```python
from build123d import *

# Parameters (mm, degrees)
SKETCH_2_W                     = 4.9
SKETCH_2_H                     = 7
EXTRUDE_1_DEPTH                = 2.7
EXTRUDE_2_DEPTH                = 0.25
FILLET_1_R                     = 0.05
CHAMFER_1_SIZE                 = 0.4
PATTERN_LINEAR_2_COUNT         = 2
PATTERN_LINEAR_2_PITCH         = 2.5
FILLET_1_OF_PATTERN_LINEAR_2_R = 0.05
MIRROR_START                   = -1.5
MIRROR_1_DEPTH                 = 0.5
MIRROR_START_2                 = 1
MIRROR_1_2_DEPTH               = 0.5
CHAMFER_2_SIZE                 = 0.4
CHAMFER_3_SIZE                 = 0.15
CHAMFER_3_SIZE2                = 0.649721381
CHAMFER_4_SIZE                 = 0.15
CHAMFER_4_SIZE2                = 0.649721381
SKETCH_7_R                     = 0.15
CUT_EXTRUDE_2_DEPTH            = 0.02
MOVE_BODY_2_ANGLE              = 120


with BuildPart() as part:
    # Эскиз2 → Бобышка-Вытянуть1 (new body)
    with BuildSketch(Plane(origin=(0, 0.15, 0), x_dir=(-1, 0, 0), z_dir=(0, 1, 0))):
        Rectangle(SKETCH_2_W, SKETCH_2_H)
    extrude(amount=EXTRUDE_1_DEPTH)

    # Эскиз4 → Вытянуть-Тонкостенный2 (add, symmetric)
    with BuildSketch(Plane(origin=(1.25, 0, 0), x_dir=(0, 0, -1), z_dir=(1, 0, 0))):
        with BuildLine():
            Line((-3.5, 1.3), (-3.905923723, 1.3))
            ThreePointArc((-3.905923723, 1.3), (-4.063504056, 1.223160215), (-4.1, 1.051684386))
            Line((-4.1, 1.051684386), (-3.9, 0.248315614))
            ThreePointArc((-3.9, 0.248315614), (-3.936495944, 0.076839785), (-4.094076277, 0))
            Line((-4.094076277, 0), (-4.6, 0))
            Line((-4.6, 0), (-4.6, 0.35))
            Line((-4.6, 0.35), (-4.285997426, 0.35))
            Line((-4.285997426, 0.35), (-4.439633485, 0.967132062))
            ThreePointArc((-4.439633485, 0.967132062), (-4.339269639, 1.438690592), (-3.905923723, 1.65))
            Line((-3.905923723, 1.65), (-3.5, 1.65))
            Line((-3.5, 1.65), (-3.5, 1.3))
        make_face()
    extrude_2 = extrude(amount=EXTRUDE_2_DEPTH, both=True)

    # Скругление1
    fillet_1_edges = [part.edges().sort_by_distance(p)[0] for p in [
        (1.25, 0.35, 4.285997426),
    ]]
    fillet(fillet_1_edges, radius=FILLET_1_R)

    # Фаска1
    chamfer_1_edges = [part.edges().sort_by_distance(p)[0] for p in [
        (0, 2.85, 3.5),
    ]]
    chamfer(chamfer_1_edges, length=CHAMFER_1_SIZE)

    # Линейный массив2: Вытянуть-Тонкостенный2 ×2
    with Locations(*[(-i * PATTERN_LINEAR_2_PITCH, 0, 0) for i in range(1, PATTERN_LINEAR_2_COUNT)]):
        add(extrude_2)

    # Скругление1 of Линейный массив2
    fillet_1_of_pattern_linear_2_edges = [part.edges().sort_by_distance(p)[0] for p in [
        (-1.25, 0.35, 4.285997426),
    ]]
    fillet(fillet_1_of_pattern_linear_2_edges, radius=FILLET_1_OF_PATTERN_LINEAR_2_R)

    # Зеркальное отражение1: read off the stored shape, not the designer's step
    # Зеркальное отражение1 outline → Зеркальное отражение1 (add)
    with BuildSketch(Plane.YZ.offset(MIRROR_START)):
        with BuildLine():
            Line((0, -4.6), (0.35, -4.6))
            Line((0.35, -4.6), (0.35, -4.349971142))
            ThreePointArc((0.35, -4.349971142), (0.369209946, -4.310576059), (0.412078903, -4.301452073))
            Line((0.412078903, -4.301452073), (0.967132062, -4.439633485))
            ThreePointArc((0.967132062, -4.439633485), (1.438690592, -4.339269639), (1.65, -3.905923723))
            Line((1.65, -3.905923723), (1.65, -3.5))
            Line((1.65, -3.5), (1.3, -3.5))
            Line((1.3, -3.5), (1.3, -3.905923723))
            ThreePointArc((1.3, -3.905923723), (1.223160215, -4.063504056), (1.051684386, -4.1))
            Line((1.051684386, -4.1), (0.248315614, -3.9))
            ThreePointArc((0.248315614, -3.9), (0.076839785, -3.936495944), (0, -4.094076277))
            Line((0, -4.094076277), (0, -4.6))
        make_face()
    extrude(amount=MIRROR_1_DEPTH)

    # Mirror 1 2 outline → Mirror 1 2 (add)
    with BuildSketch(Plane.YZ.offset(MIRROR_START_2)):
        with BuildLine():
            Line((0, -4.6), (0.35, -4.6))
            Line((0.35, -4.6), (0.35, -4.349971142))
            ThreePointArc((0.35, -4.349971142), (0.369209946, -4.310576059), (0.412078903, -4.301452073))
            Line((0.412078903, -4.301452073), (0.967132062, -4.439633485))
            ThreePointArc((0.967132062, -4.439633485), (1.438690592, -4.339269639), (1.65, -3.905923723))
            Line((1.65, -3.905923723), (1.65, -3.5))
            Line((1.65, -3.5), (1.3, -3.5))
            Line((1.3, -3.5), (1.3, -3.905923723))
            ThreePointArc((1.3, -3.905923723), (1.223160215, -4.063504056), (1.051684386, -4.1))
            Line((1.051684386, -4.1), (0.248315614, -3.9))
            ThreePointArc((0.248315614, -3.9), (0.076839785, -3.936495944), (0, -4.094076277))
            Line((0, -4.094076277), (0, -4.6))
        make_face()
    extrude(amount=MIRROR_1_2_DEPTH)

    # Фаска2
    chamfer_2_edges = [part.edges().sort_by_distance(p)[0] for p in [
        (0, 2.85, -3.5),
    ]]
    chamfer(chamfer_2_edges, length=CHAMFER_2_SIZE)

    # Фаска3
    chamfer_3_edges = [part.edges().sort_by_distance(p)[0] for p in [
        (0, 0.15, -3.5),
    ]]
    chamfer_3_side = [part.faces().sort_by_distance(p)[0] for p in [
        (0, 0.15, 0),
    ]]
    chamfer(chamfer_3_edges, length=CHAMFER_3_SIZE, length2=CHAMFER_3_SIZE2, reference=chamfer_3_side[0])

    # Фаска4
    chamfer_4_edges = [part.edges().sort_by_distance(p)[0] for p in [
        (0, 0.15, 3.5),
    ]]
    chamfer_4_side = [part.faces().sort_by_distance(p)[0] for p in [
        (0, 0.15, 0.075),
    ]]
    chamfer(chamfer_4_edges, length=CHAMFER_4_SIZE, length2=CHAMFER_4_SIZE2, reference=chamfer_4_side[0])

    # Эскиз7 → Вырез-Вытянуть2 (cut)
    with BuildSketch(Plane(origin=(0, 2.85, 0), x_dir=(1, 0, 0), z_dir=(0, 1, 0))):
        with Locations(Location((-1.95, -2.8, 0), (0, 0, 270))):
            Circle(SKETCH_7_R)
    extrude(amount=-CUT_EXTRUDE_2_DEPTH, mode=Mode.SUBTRACT)


with BuildPart() as part_1:
    # Move Body 2: read off the stored shape, not the designer's step
    # Move Body 2: moved
    add(part.part.moved(Location((1.25, 0, -4.425))).rotate(Axis((0, 0, 0), (0.5773502692, -0.5773502692, -0.5773502692)), MOVE_BODY_2_ANGLE))


solid = part_1.part
```
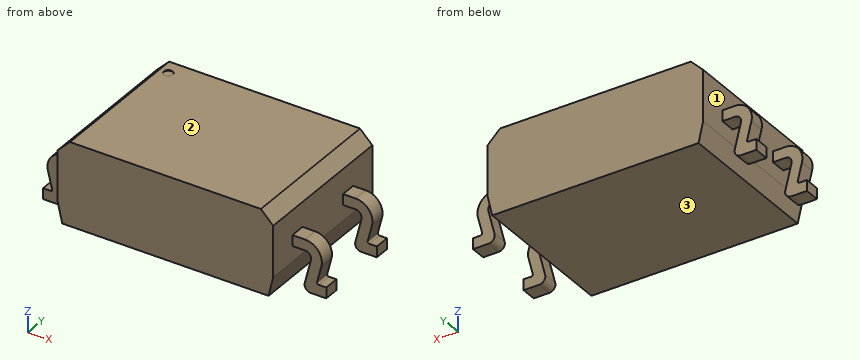
Can you work these out from the model? Positions are in its coordinate system, mm. Face numbers are marked on the shaded views. Give positions to 0.01 mm unless a question says otherwise; leave off trailing zeros. Order: outer loops, then holes, each group sorted by start corner. A loop starts at its lowest first (then second) coordinate and runs counter-clockwise, first axis right, second up. Notation, with made-up numbers: M -27,-19.5 L 1,-19.5 A13 ccw 1,-0.5 Z; hole C 29,27.5 d1. An arc over 180 degrees is marked long. Write item = value, one per line. Start each with the question number.
Q1. Suppose I cut it at A-A (y = -2.15). Write out the boundary of the cut face in (x, z) (3 decimals).
Q2. Suppose I cut it at D-D (y = 0.7). Write out the boundary of the cut face in (x, z) (3 decimals), plus the area to 3 significant figures.
Q3. We'd pull the mould along Z, two halves only. Please class the marked faces 1, 2 and 3: pulls with the +Z half, pulls with the -Z half, needs draft (parallel to the pull), parting line crosses it, or undercut.
Q4. Suppose I cut it at B-B (z = 1.15). Write out the boundary of the cut face in (x, y) (3 decimals), plus the area to 3 significant figures.
Q5. Will these pins go through, and if not, where does the flat tip stop? pin 1 Ø0.9 at (x, z) = (8.5, 0.5) entering from -Y; pin 2 Ø0.9 at (x, z) = (0.5, 0.5) entering from +Y; pin 3 Ø1.3 at (y, z) = (-2.5, 1.5) entering from -X; pin 4 Ø1.2 at (x, z) = (8, 1) entering from -Y.
Q6. Suppose I cut it at C-C (x = 2.25). Write out the boundary of the cut face in (y, z).
Q7. I need wall thicknesses on probe 1 along Z at (x, y) = (7, 0.8); probe 2 along X at (y, z) = (-1.9, 1.35) (3 decimals); probe 3 along X at (y, z) = (-2.7, 1) (3 decimals). Which ranges of each line are inside material? Lowest first, please. Write a range as [from, to].
Check result:
q1.outline = M 0.925,0.8 L 1.075,0.15 L 7.775,0.15 L 7.925,0.8 L 7.925,2.45 L 7.525,2.85 L 1.325,2.85 L 0.925,2.45 Z
q2.outline = M 0.925,0.8 L 1.075,0.15 L 7.775,0.15 L 7.925,0.8 L 7.925,2.45 L 7.525,2.85 L 1.775,2.85 L 1.775,2.83 L 1.475,2.83 L 1.475,2.85 L 1.325,2.85 L 0.925,2.45 Z
q2.area = 18.6 mm2
q3.face_1 = needs draft
q3.face_2 = pulls with the +Z half
q3.face_3 = pulls with the -Z half
q4.outline = M -0.029,-2.75 L 0.325,-2.75 L 0.325,-2.25 L -0.029,-2.25 Z; M -0.029,-0.25 L 0.325,-0.25 L 0.325,0.25 L -0.029,0.25 Z; M 0.925,-3.7 L 7.925,-3.7 L 7.925,1.2 L 0.925,1.2 Z; M 8.525,-2.75 L 8.879,-2.75 L 8.879,-2.25 L 8.525,-2.25 Z; M 8.525,-0.25 L 8.879,-0.25 L 8.879,0.25 L 8.525,0.25 Z
q4.area = 35.0 mm2
q5.pin_1 = -2.75
q5.pin_2 = 0.25
q5.pin_3 = -0.03
q5.pin_4 = -3.7
q6.outline = M -3.7,0.15 L 1.2,0.15 L 1.2,2.85 L -3.7,2.85 Z
q7.probe_1 = [0.15, 2.85]
q7.probe_2 = [0.925, 7.925]
q7.probe_3 = [-0.022, 0.338], [0.925, 7.925], [8.512, 8.872]
